from build123d import *

# Parameters (mm, degrees)
SKETCH_W  = 450
SKETCH_H  = 250
SKETCH_R  = 25
PAD_DEPTH = 6


with BuildPart() as part:
    # Sketch → Pad (new body)
    with BuildSketch(Plane.YZ):
        with Locations((225, 125)):
            Rectangle(SKETCH_W, SKETCH_H)
        with Locations((132, 147)):
            Circle(SKETCH_R, mode=Mode.SUBTRACT)
    extrude(amount=PAD_DEPTH)


solid = part.part
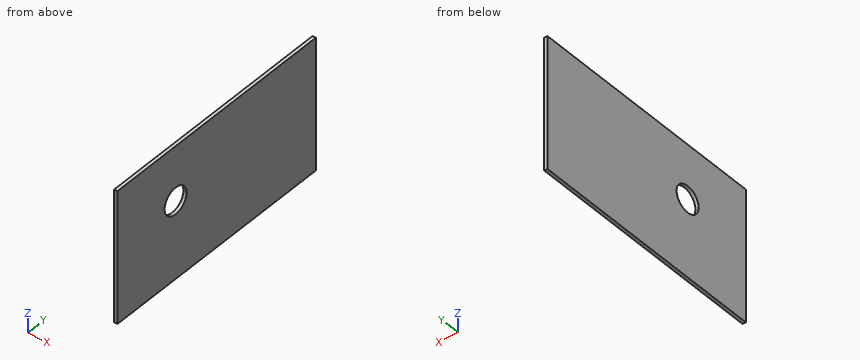
CAD build for the part. Positions are in the model's coordinates, mm. Coordinates: 2 decimals unless noted, no trailing zeros. Write each loop counter-clockwise with the first axis right and the second up, starting at its lowest first coordinate (ties: lowest second). Pieces come first, ordered by that corner, then holes. Notation, with made-up numbers: M 13.5,9 L 21.5,9 A36 cw 21.5,47 Z; hole C 27.5,-5.75 d3. An arc over 180 degrees is marked long. Return JSON: item names as keys, results as strings.
Item 1: Slice it at B-B, the plane z = 147. Write the cut outline in (x, y), and give its area (3 significant figures).
Findings below:
{"outline": "M 0,0 L 6,0 L 6,107 L 0,107 Z; M 0,157 L 6,157 L 6,450 L 0,450 Z", "area": "2,400 mm2"}
Item 2: Slice it at C-C, the plane y = 132. Write the cut outline in (x, z), and give its area (3 significant figures).
Findings below:
{"outline": "M 0,0 L 6,0 L 6,122 L 0,122 Z; M 0,172 L 6,172 L 6,250 L 0,250 Z", "area": "1,200 mm2"}
Item 3: Drop a flat-ended pin along its axis: pin 1 Ø2 at (y, z) = (175.5, 142.5) entering from -X. Give the stop position or say it passes through.
Findings below:
{"pin 1": "stops at x = 0"}
Item 4: Slice it at A-A, the plane x = 1.8. Write the cut outline in (y, z), and give its area (3 significant figures).
Findings below:
{"outline": "M 0,0 L 450,0 L 450,250 L 0,250 Z; hole C 132,147 d50", "area": "111,000 mm2"}
Item 5: Probe line 1 (Z direction, x = 3.9, y = 132); line 2 (Y direction, x = 2.35, z = 130); line 3 (Z direction, x = 5.75, y = 125). List the from-to ranges inside material, lowest first. Write a range as from..to.
Findings below:
{"line 1": "z = 0..122, 172..250", "line 2": "y = 0..113.67, 150.33..450", "line 3": "z = 0..123, 171..250"}
